```python
from build123d import *

# Parameters (mm, degrees)
BOSS_EXTRUDE1_DEPTH = 30
SKETCH2_R           = 4
SKETCH2_R_2         = 1.75
CUT_EXTRUDE1_DEPTH  = 83.800966178


with BuildPart() as part:
    # Sketch1 → Boss-Extrude1 (new body)
    with BuildSketch(Plane(origin=(0, 0, 0), x_dir=(1, 0, 0), z_dir=(0, 1, 0))):
        Polygon((0, 0), (0, 66), (40, 66), (40, 63), (3, 63), (3, 3), (40, 3), (40, 0), align=None)
    extrude(amount=BOSS_EXTRUDE1_DEPTH)

    # Sketch2 → Cut-Extrude1 (cut, through all)
    with BuildSketch(Plane.XY):
        with Locations((27.5, 15)):
            Circle(SKETCH2_R)
        with Locations((19.5, 15)):
            Circle(SKETCH2_R_2)
        with Locations((27.5, 23)):
            Circle(SKETCH2_R_2)
        with Locations((35.5, 15)):
            Circle(SKETCH2_R_2)
        with Locations((27.5, 7)):
            Circle(SKETCH2_R_2)
    extrude(amount=-CUT_EXTRUDE1_DEPTH, mode=Mode.SUBTRACT)


solid = part.part
```
The model under review builds one solid part; all positions refer to its coordinate system, in mm. A direction names the side the tool comes from. Round coordinates to 2 decimals unless told otherwise and drop trailing zeros. Loops run counter-clockwise (first coordinate to the right, second up) from the corner with the lowest first, then second, coordinate; pieces in that order, holes last. Notation, with made-up numbers: M -32,-37 L 25,-37 A11 ccw 25,-28 Z; hole C 86.5,4.5 d10. An arc over 180 degrees is marked long. Put each result on its own line as item: value.
Q1. Consider section C-C, the plane x = 19.5. Give the boundary of the cut face in (y, z).
Result set:
outline: M 0,-66 L 13.25,-66 L 13.25,-63 L 0,-63 Z; M 0,-3 L 13.25,-3 L 13.25,0 L 0,0 Z; M 16.75,-66 L 30,-66 L 30,-63 L 16.75,-63 Z; M 16.75,-3 L 30,-3 L 30,0 L 16.75,0 Z
Q2. Consider section D-D, the plane x = 27.5. Count the separate pieces of the cut face and the enclosed holes in it, then the cut area to 3 significant figures.
Result set:
separate pieces: 8
enclosed holes: 0
area: 90.0 mm²
Q3. Consider section A-A, the plane y = 7. Give the boundary of the cut face in (x, z).
Result set:
outline: M 0,-66 L 25.75,-66 L 25.75,-63 L 3,-63 L 3,-3 L 25.75,-3 L 25.75,0 L 0,0 Z; M 29.25,-66 L 40,-66 L 40,-63 L 29.25,-63 Z; M 29.25,-3 L 40,-3 L 40,0 L 29.25,0 Z
Q4. For pin 1 (1 mm diameter, centred on y = 16.5, z = -7.5, fed in from +X); pin 2 (2 mm diameter, centred on x = 27.5, y = 7, fed in from -Z), all flat-tipped, find the tip position at first contact; note any pin that passes through.
Result set:
pin 1: stops at x = 3
pin 2: passes through
Q5. Machinability: for faces 1 (the cylindrical face through (25.75, 7.08, -64.48)), 2 (the flat face through (21, 11, -3)), which of the approach directions +Z, -Z, +X, -X, +Y, -Y give a long, thin tool a straight path to every point of the face, cutting with its end or side? Answer none if there is none.
Result set:
face 1: +Z, -Z
face 2: +X, +Y, -Y
Q6. Mouldability with a two-part tool opening along Y and no side actions: class faces 3 (the flat face through (0, 15, -33)), 4 (the cylindrical face through (24.55, 17.7, -64.48)), 5 (the flat face through (2, 0, -33)) as released by +Y, released by -Y, zero draft, split by the parting line, or undercut.
Result set:
face 3: zero draft
face 4: undercut
face 5: released by -Y
Q7. To check wall thickness, follow L1, parallel to Y at x = 27.5, z = -1; L2, parallel to Z at x = 35.5, y = 23.5; L3, parallel to Y at x = 35.5, z = -64.45. State the ranges of each line that lie inside material, in increasing order.
Result set:
L1: y = 0 to 5.25, 8.75 to 11, 19 to 21.25, 24.75 to 30
L2: z = -66 to -63, -3 to 0
L3: y = 0 to 13.25, 16.75 to 30
Q8. Consider section B-B, the plane x = 14. Give the boundary of the cut face in (y, z), then the cut area to 3 significant figures.
Result set:
outline: M 0,-66 L 30,-66 L 30,-63 L 0,-63 Z; M 0,-3 L 30,-3 L 30,0 L 0,0 Z
area: 180 mm²
